Build history of the part. All positions in model axes, mm. Face numbers are marked on the shaded views. A direction names the side the tool comes from. Coordinates: 2 decimals unless noted, no trailing zeros. Loops run counter-clockwise (first coordinate to the right, second up) from the corner with the lowest first, then second, coordinate; pieces in that order, holes last.
(1) Tool access for the marked faces 1 and 2: list every direction of +Z, -Z, +X, -X, +Y, -Y with a clear straight run to the whole face (end or side of a thin tool).
(2) Slice it at D-D (z = 2.75). Give the cut face in (x, y).
(3) Slice it at A-A (y = -21.5). Give the cut face in (x, z).
(4) Slice it at C-C (x = 1.5). Give the cut face in (y, z).
(5) Flat gauge pins, fed straight in: P1, Ø2, axis at y = -35, z = -2, coming from the -X side; P2, Ø2.5, axis at x = 0, y = 9.25, coming from the +Z side; P3, Ø0.7, axis at x = 4.5, y = -31.5, coming from the +Z side; P4, Ø0.6, axis at y = -18, z = -4.5, coming from the +X side. Where does each tip first touch, or does it go through?
(6) Wall check: L1, parallel to Y at x = 0, z = -4.25; L2, parallel to Y at x = 0, z = -5.5; L3, parallel to X at y = -23.5, z = -0.25. Give the ranges that are in metal, low to high.
(7) Slice it at B-B (z = 0). Give the cut face in (x, y), and give its area (3 significant figures).
from build123d import *

# Parameters (mm, degrees)
SKETCH1_R               = 6
BOSS_EXTRUDE1_DEPTH     = 12
CUT_EXTRUDE1_DEPTH      = 15.696938457
CUT_EXTRUDE1_DEPTH_BACK = 15.696938457
SKETCH2_W               = 7.5
SKETCH2_H               = 8.5
CUT_EXTRUDE2_DEPTH      = 15.696938457
CUT_EXTRUDE2_DEPTH_BACK = 15.696938457
SKETCH3_R               = 0.75
BOSS_EXTRUDE2_START     = 42
SKETCH4_R               = 6
BOSS_EXTRUDE2_DEPTH     = 42


with BuildPart() as part:
    # Sketch1 → Boss-Extrude1 (new body)
    with BuildSketch(Plane(origin=(0, 0, 0), x_dir=(1, 0, 0), z_dir=(0, 1, 0))):
        with Locations(Location((0, 0, 0), (0, 0, 270))):
            Circle(SKETCH1_R)
    extrude(amount=BOSS_EXTRUDE1_DEPTH)

    # Sketch2 → Cut-Extrude1 (cut, two sides: drawn at the far end of the back side and taken through both)
    with BuildSketch(Plane(origin=(0, 0, 0), x_dir=(0, 0, -1), z_dir=(1, 0, 0)).offset(-CUT_EXTRUDE1_DEPTH_BACK)):
        with Locations((0, 7.75)):
            Rectangle(SKETCH2_W, SKETCH2_H)
    extrude(amount=CUT_EXTRUDE1_DEPTH + CUT_EXTRUDE1_DEPTH_BACK, mode=Mode.SUBTRACT)

    # Sketch3 → Cut-Extrude2 (cut, two sides: drawn at the far end of the back side and taken through both)
    with BuildSketch(Plane.XY.offset(-CUT_EXTRUDE2_DEPTH_BACK)):
        with BuildLine():
            Line((-3.15, 5), (-3.15, 8.85))
            ThreePointArc((-3.15, 8.85), (-2.227386361, 11.077386361), (0, 12))
            Line((0, 12), (-4.683748499, 12))
            Line((-4.683748499, 12), (-4.683748499, 3.5))
            Line((-4.683748499, 3.5), (-4.65, 3.5))
            ThreePointArc((-4.65, 3.5), (-3.589339828, 3.939339828), (-3.15, 5))
        make_face()
        with BuildLine():
            Line((4.683748499, 12), (0, 12))
            ThreePointArc((0, 12), (2.227386361, 11.077386361), (3.15, 8.85))
            Line((3.15, 8.85), (3.15, 5))
            ThreePointArc((3.15, 5), (3.589339828, 3.939339828), (4.65, 3.5))
            Line((4.65, 3.5), (4.683748499, 3.5))
            Line((4.683748499, 3.5), (4.683748499, 12))
        make_face()
        with Locations((0, 9.25)):
            Circle(SKETCH3_R)
    extrude(amount=CUT_EXTRUDE2_DEPTH + CUT_EXTRUDE2_DEPTH_BACK, mode=Mode.SUBTRACT)

    # Sketch4 → Boss-Extrude2 (add)
    with BuildSketch(Plane.XZ.offset(BOSS_EXTRUDE2_START)):
        with Locations(Location((0, 0, 0), (0, 0, 270))):
            Circle(SKETCH4_R)
        with BuildLine():
            Line((-0.6, 4.207433897), (-0.6, 5))
            Line((-0.6, 5), (0.6, 5))
            Line((0.6, 5), (0.6, 4.207433897))
            ThreePointArc((0.6, 4.207433897), (2.799894973, 3.19735643), (4.091454509, 1.15))
            Line((4.091454509, 1.15), (5, 1.15))
            Line((5, 1.15), (5, -1.15))
            Line((5, -1.15), (4.091454509, -1.15))
            ThreePointArc((4.091454509, -1.15), (2.799894973, -3.19735643), (0.6, -4.207433897))
            Line((0.6, -4.207433897), (0.6, -5))
            Line((0.6, -5), (-0.6, -5))
            Line((-0.6, -5), (-0.6, -4.207433897))
            ThreePointArc((-0.6, -4.207433897), (-2.799894973, -3.19735643), (-4.091454509, -1.15))
            Line((-4.091454509, -1.15), (-5, -1.15))
            Line((-5, -1.15), (-5, 1.15))
            Line((-5, 1.15), (-4.091454509, 1.15))
            ThreePointArc((-4.091454509, 1.15), (-2.799894973, 3.19735643), (-0.6, 4.207433897))
        make_face(mode=Mode.SUBTRACT)
    extrude(amount=-BOSS_EXTRUDE2_DEPTH)


solid = part.part
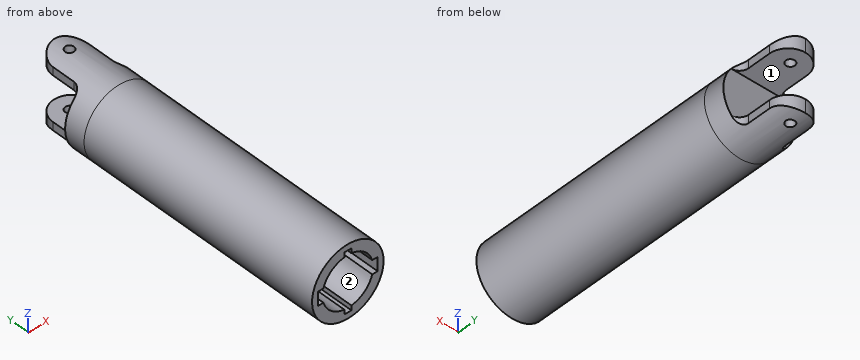
Response values:
1. face 1: +X, -X, +Y
1. face 2: -Y
2. outline: (-5.33, -42) - (-3.24, -42) - (-3.24, 0) - (3.24, 0) - (3.24, -42) - (5.33, -42) - (5.33, 3.5) - (-5.33, 3.5) - close
3. outline: circle Ø12 at (0, 0); hole (-5, -1.15) - (-4.09, -1.15) arc R4.25 ccw to (-0.6, -4.21) - (-0.6, -5) - (0.6, -5) - (0.6, -4.21) arc R4.25 ccw to (4.09, -1.15) - (5, -1.15) - (5, 1.15) - (4.09, 1.15) arc R4.25 ccw to (0.6, 4.21) - (0.6, 5) - (-0.6, 5) - (-0.6, 4.21) arc R4.25 ccw to (-4.09, 1.15) - (-5, 1.15) - close
4. outline: (-42, -5.81) - (11.62, -5.81) - (11.62, -3.75) - (3.5, -3.75) - (3.5, 3.75) - (11.62, 3.75) - (11.62, 5.81) - (-42, 5.81) - (-42, 3.98) - (0, 3.98) - (0, -3.98) - (-42, -3.98) - close
5. P1: stops at x = -5.92
5. P2: stops at z = 6
5. P3: stops at z = 4.33
5. P4: stops at x = 4.28
6. L1: y = 0 to 8.5, 10 to 12
6. L2: y = -42 to 8.5, 10 to 12
6. L3: x = -5.99 to -5, 5 to 5.99
7. outline: (-6, -42) - (-5, -42) - (-5, 0) - (5, 0) - (5, -42) - (6, -42) - (6, 3.5) - (-6, 3.5) - close
7. area: 126 mm2
